Could you check a few things on this model? Use its own coordinates, in mm. A direction names the side the tool comes from. Coordinates: 2 decimals unless noted, no trailing zeros. Loops run counter-clockwise (first coordinate to the right, second up) from the corner with the lowest first, then second, coordinate; pieces in that order, holes last. Notation, with made-up numbers: (-18.75, -33.75) - (-3.75, -33.75) arc R30 ccw to (-3.75, 2.25) - close; hole circle Ø9 at (-32, 32). An arc over 180 degrees is marked (long way). Put each result on its own line as item: value. Start each with the question number.
```python
from build123d import *

# Parameters (mm, degrees)
ESQUISSE1_W              = 140
ESQUISSE1_H              = 340
ESQUISSE1_R              = 1.5
ESQUISSE1_W_2            = 30
ESQUISSE1_H_2            = 6
BOSS_EXTRU_3_DEPTH       = 6
ESQUISSE4_W              = 6
ESQUISSE4_H              = 28
ESQUISSE4_H_2            = 85
ESQUISSE4_H_3            = 51
ESQUISSE4_H_4            = 21
ENL_V_MAT_EXTRU_2_DEPTH  = 6
ESQUISSE5_R              = 1.5
ENL_V_MAT_EXTRU_3_DEPTH  = 9
ENL_V_START              = -3
ESQUISSE6_R              = 1.5
ENL_V_MAT_EXTRU_6_DEPTH  = 3
ESQUISSE7_W              = 20
ESQUISSE7_H              = 6
ENL_V_MAT_EXTRU_7_DEPTH  = 10
ENL_V_MAT_EXTRU_8_DEPTH  = 6
ESQUISSE9_W              = 40
ESQUISSE9_H              = 6
ENL_V_MAT_EXTRU_9_DEPTH  = 6
ESQUISSE10_R             = 1.5
ESQUISSE10_W             = 30
ESQUISSE10_H             = 6
ENL_V_MAT_EXTRU_10_DEPTH = 6


with BuildPart() as part:
    # Esquisse1 → Boss.-Extru.3 (new body)
    with BuildSketch(Plane.XY):
        with Locations((69.996437878, -101.21224042)):
            Rectangle(ESQUISSE1_W, ESQUISSE1_H)
        with Locations((14.996437878, 65.78775958)):
            Circle(ESQUISSE1_R, mode=Mode.SUBTRACT)
        with Locations((124.996437878, 65.78775958)):
            Circle(ESQUISSE1_R, mode=Mode.SUBTRACT)
        with Locations((69.996437878, 65.78775958)):
            Circle(ESQUISSE1_R, mode=Mode.SUBTRACT)
        with Locations((22.996437878, -112.21224042)):
            Circle(ESQUISSE1_R, mode=Mode.SUBTRACT)
        with Locations((116.996437878, -112.21224042)):
            Circle(ESQUISSE1_R, mode=Mode.SUBTRACT)
        with Locations((69.996437878, -112.21224042)):
            Rectangle(ESQUISSE1_W_2, ESQUISSE1_H_2, mode=Mode.SUBTRACT)
    extrude(amount=BOSS_EXTRU_3_DEPTH)

    # Esquisse4 → Enlèv. mat.-Extru.2 (cut)
    with BuildSketch(Plane.XY):
        with Locations((2.996437878, 54.78775958)):
            Rectangle(ESQUISSE4_W, ESQUISSE4_H)
        with Locations((2.996437878, -31.71224042)):
            Rectangle(ESQUISSE4_W, ESQUISSE4_H_2)
        with Locations((2.996437878, -129.71224042)):
            Rectangle(ESQUISSE4_W, ESQUISSE4_H_3)
        with Locations((136.996437878, -114.71224042)):
            Rectangle(ESQUISSE4_W, ESQUISSE4_H_4)
        with Locations((136.996437878, -31.71224042)):
            Rectangle(ESQUISSE4_W, ESQUISSE4_H_2)
        with Locations((136.996437878, 54.78775958)):
            Rectangle(ESQUISSE4_W, ESQUISSE4_H)
    extrude(amount=ENL_V_MAT_EXTRU_2_DEPTH, mode=Mode.SUBTRACT)

    # Esquisse5 → Enlèv. mat.-Extru.3 (cut)
    with BuildSketch(Plane(origin=(0, 0, 0), x_dir=(0, 0, -1), z_dir=(1, 0, 0))):
        with Locations(Location((-3, -126.71224042, 0), (0, 0, 270))):
            Circle(ESQUISSE5_R)
        with Locations(Location((-3, -51.71224042, 0), (0, 0, 270))):
            Circle(ESQUISSE5_R)
        with Locations(Location((-3, -6.21224042, 0), (0, 0, 270))):
            Circle(ESQUISSE5_R)
        with Locations(Location((-3, 57.78775958, 0), (0, 0, 270))):
            Circle(ESQUISSE5_R)
    extrude(amount=ENL_V_MAT_EXTRU_3_DEPTH, mode=Mode.SUBTRACT)

    # Esquisse6 → Enlèv. mat.-Extru.6 (cut)
    with BuildSketch(Plane(origin=(133.996437878, 0, 0), x_dir=(0, 0, -1), z_dir=(1, 0, 0)).offset(ENL_V_START)):
        with Locations(Location((-3, -6.21224042, 0), (0, 0, 270))):
            Circle(ESQUISSE6_R)
        with Locations(Location((-3, -51.71224042, 0), (0, 0, 270))):
            Circle(ESQUISSE6_R)
        with Locations(Location((-3, 57.78775958, 0), (0, 0, 270))):
            Circle(ESQUISSE6_R)
    extrude(amount=ENL_V_MAT_EXTRU_6_DEPTH, mode=Mode.SUBTRACT)

    # Esquisse7 → Enlèv. mat.-Extru.7 (cut)
    with BuildSketch(Plane.XY):
        with Locations((129.996437878, -268.21224042)):
            Rectangle(ESQUISSE7_W, ESQUISSE7_H)
        with Locations((89.996437878, -268.21224042)):
            Rectangle(ESQUISSE7_W, ESQUISSE7_H)
    extrude(amount=ENL_V_MAT_EXTRU_7_DEPTH, mode=Mode.SUBTRACT)

    # Esquisse8 → Enlèv. mat.-Extru.8 (cut)
    with BuildSketch(Plane.XY.offset(6)):
        with BuildLine():
            Line((79.996437878, -265.21224042), (79.996437878, -200.21224042))
            ThreePointArc((79.996437878, -200.21224042), (42.996437878, -187.445703134), (5.996437878, -200.21224042))
            Line((5.996437878, -200.21224042), (5.996437878, -155.21224042))
            Line((5.996437878, -155.21224042), (-0.003562122, -155.21224042))
            Line((-0.003562122, -155.21224042), (-0.003562122, -271.21224042))
            Line((-0.003562122, -271.21224042), (79.996437878, -271.21224042))
            Line((79.996437878, -271.21224042), (79.996437878, -265.21224042))
        make_face()
    extrude(amount=-ENL_V_MAT_EXTRU_8_DEPTH, mode=Mode.SUBTRACT)

    # Esquisse9 → Enlèv. mat.-Extru.9 (cut)
    with BuildSketch(Plane.XY.offset(6)):
        with Locations((39.996437878, 65.78775958)):
            Rectangle(ESQUISSE9_W, ESQUISSE9_H)
        with Locations((99.996437878, 65.78775958)):
            Rectangle(ESQUISSE9_W, ESQUISSE9_H)
    extrude(amount=-ENL_V_MAT_EXTRU_9_DEPTH, mode=Mode.SUBTRACT)

    # Esquisse10 → Enlèv. mat.-Extru.10 (cut)
    with BuildSketch(Plane(origin=(0, 0, 0), x_dir=(-1, 0, 0), z_dir=(0, 0, -1))):
        with Locations((-116.996437878, -56.21224042)):
            Circle(ESQUISSE10_R)
        with Locations((-22.996437878, -56.21224042)):
            Circle(ESQUISSE10_R)
        with Locations((-69.996437878, -56.21224042)):
            Rectangle(ESQUISSE10_W, ESQUISSE10_H)
    extrude(amount=-ENL_V_MAT_EXTRU_10_DEPTH, mode=Mode.SUBTRACT)


solid = part.part
```
(1) I want a section at D-D on x = 51. List the corners of the cut face in (y, z) for me.
(2) Which directions (+Z, -Z, +X, -X, +Y, -Y) give clear straight access to the entire face, cutting with the end or side of a thin tool? Please do faces 1 (the flat face through (119.996, -268, 3)), 2 (the flat face through (137, 40.788, 3)), 3 (the flat face through (3, 10.788, 3)).
(3) I want a section at B-B on y = -152. List the corners of the cut face in (x, z) for me.
(4) For pin 1 Ø1 at (y, z) = (-59, 0.5) entering from -X; pin 2 Ø1.8 at (y, z) = (57.79, 3) entering from -X; pin 3 Ø1.8 at (y, z) = (-267.5, 2) entering from +X, each with a flat end and sliding along its axis, tell me the tip position at first contact or that it passes through.
(5) I need wall thicknesses on L1, parallel to Y at x = 117, z = 2.9; L2, parallel to Y at x = 74, z = 0.35; L3, parallel to Y at x = 8.5, z = 3.55. Which ranges of each line are inside material? Lowest first, please. Write a range as [from, to].
(6) If we mould it in two halves opening along Y, with no side actions, what happens to faces 4 (the cylindrical face through (43.55, -187.45, 3.04)), 5 (the flat face through (79.996, 66, 3)), 6 (the flat face through (137, -74.212, 3))? For each: pulls with the +Y half, pulls with the -Y half, needs draft (parallel to the pull), parting line crosses it, or undercut.
(7) I want a section at C-C on z = 3. Count the separate pieces of the cut face and the enclosed holes in it, and give its area (3 significant figures).
(8) I want a section at A-A on x = 76. List the corners of the cut face in (y, z) for me, and give its area (3 significant figures).
Answer sheet:
1. outline: (-187.98, 0) - (62.79, 0) - (62.79, 6) - (-187.98, 6) - close
2. face 1: +Z, -Z, +X, -Y
2. face 2: +Z, -Z, +X, +Y
2. face 3: +Z, -Z, -X
3. outline: (6, 0) - (140, 0) - (140, 6) - (6, 6) - close
4. pin 1: stops at x = 6
4. pin 2: stops at x = 9
4. pin 3: stops at x = 120
5. L1: y = [-271.21, -113.71], [-110.71, -57.71], [-54.71, 62.79]
5. L2: y = [-196.08, -115.21], [-109.21, -59.21], [-53.21, 68.79]
5. L3: y = [-198.35, -128.11], [-125.32, -53.11], [-50.32, -7.61], [-4.82, 56.39], [59.18, 68.79]
6. face 4: pulls with the -Y half
6. face 5: needs draft
6. face 6: undercut
7. separate pieces: 1
7. enclosed holes: 9
7. area: 38,000 mm^2
8. outline: (-197.34, 0) - (-115.21, 0) - (-115.21, 6) - (-197.34, 6) - close; (-109.21, 0) - (-59.21, 0) - (-59.21, 6) - (-109.21, 6) - close; (-53.21, 0) - (68.79, 0) - (68.79, 6) - (-53.21, 6) - close
8. area: 1,520 mm^2
